Autodesk Inventor part; units mm, degrees
ref_plane "YZ Plane" through (0, 0, 0) normal (1, 0, 0) x (0, 1, 0)
ref_plane "XZ Plane" through (0, 0, 0) normal (0, 1, 0) x (-1, 0, 0)
ref_plane "XY Plane" through (0, 0, 0) normal (0, 0, 1) x (1, 0, 0)
sketch "Szkic1" plane through (0, 0, 0) normal (0, 0, 1) x (1, 0, 0)
  line L0 (0, 0) -> (50, 0) construction
  line L1 (50, 0) -> (50, 18) construction
  line L2 (50, 18) -> (0, 18) construction
  line L3 (0, 18) -> (0, 0) construction
  line L4 (25, 18) -> (25, 0) construction
  line L5 (0, 0) -> (0, 6) construction
  line L6 (0, 6) -> (50, 6) construction
  line L7 (50, 6) -> (50, 12) construction
  line L8 (50, 12) -> (0, 12) construction
  line L9 (0, 12) -> (0, 6) construction
  line L10 (0, 18) -> (10, 18) construction
  line L11 (10, 18) -> (10, 0) construction
  line L12 (50, 18) -> (30, 18) construction
  line L13 (30, 18) -> (30, 0) construction
  line L14 (40, 18) -> (40, 0) construction
  line L15 (0, 0) -> (50, 0)
  line L16 (50, 0) -> (50, 18)
  line L17 (50, 18) -> (40, 18)
  line L18 (40, 18) -> (40, 6)
  line L19 (40, 6) -> (10, 6)
  line L20 (10, 6) -> (10, 12)
  line L21 (10, 12) -> (30, 12)
  line L22 (30, 12) -> (30, 18)
  line L23 (30, 18) -> (0, 18)
  line L24 (0, 18) -> (0, 0)
  dimension "d1" = 18
  dimension "d2" = 6
  dimension "d3" = 6
  dimension "d4" = 10
  dimension "d5" = 20
  dimension "d8" = 20
extrude "Wyciągnięcie proste1" add sketch "Szkic1" along normal blind 6
properties part number "Zamkek_puszka"
Check sheet for the modelled part. Datum: model origin and axes. Units: mm. A direction names the side the tool comes from. Round coordinates to 2 decimals unless told otherwise and drop trailing zeros. Order: outer loops, then holes, each group sorted by start corner. A loop starts at its lowest first (then second) coordinate and runs counter-clockwise, first axis right, second up. Notation, with made-up numbers: (44.25, 85.25) -> (75.25, 85.25) arc R14 cw to (75.25, 107.25) -> close; hole circle Ø11 at (71.5, 35.25). An arc over 180 degrees is marked (long way). Use CSV: the item, a comma, the result in double quotes.
(1) Cross-section at B-B (z = 3.55). Record the boundary of the cut face in (x, y), and give its area (3 significant figures).
Worked out:
outline,"(0, 0) -> (50, 0) -> (50, 18) -> (40, 18) -> (40, 6) -> (10, 6) -> (10, 12) -> (30, 12) -> (30, 18) -> (0, 18) -> close"
area,"660 mm²"
(2) Draft check along X on faces 1 (the face through (50, 9, 3)), 2 (the face through (0, 9, 3)), 3 (the face through (15, 18, 3)), 4 (the face through (25, 6, 3)). Enter one of: pulls with the +X half, pulls with the -X half, needs draft (parallel to the pull), parting line crosses it, or undercut.
Worked out:
face 1,"pulls with the +X half"
face 2,"pulls with the -X half"
face 3,"needs draft"
face 4,"undercut"
(3) Cross-section at A-A (y = 13). Record the boundary of the cut face in (x, z).
Worked out:
outline,"(0, 0) -> (30, 0) -> (30, 6) -> (0, 6) -> close; (40, 0) -> (50, 0) -> (50, 6) -> (40, 6) -> close"
(4) Tool access check on faces 5 (the face through (20, 12, 3)), 6 (the face through (25, 5, 6)), 7 (the face through (30, 15, 3)). Record the directions out of +Z, -Z, +X, -X, +Y, -Y that give a thin tool (end or side, any length) a straight path to the whole face; none if there is none.
Worked out:
face 5,"+Z, -Z"
face 6,"+Z, +X, -X, +Y, -Y"
face 7,"+Z, -Z, +Y"
(5) Cross-section at C-C (x = 15). Record the boundary of the cut face in (y, z).
Worked out:
outline,"(0, 0) -> (6, 0) -> (6, 6) -> (0, 6) -> close; (12, 0) -> (18, 0) -> (18, 6) -> (12, 6) -> close"
(6) Material ranges on line 1 along X through (y, z) = (16.5, 2.1); line 2 along X through (y, z) = (9, 0.4); line 3 along Y through (x, z) = (29.5, 3.3), recorded low to high. Write a range as from..to.
Worked out:
line 1,"0..30, 40..50"
line 2,"0..10, 40..50"
line 3,"0..6, 12..18"
(7) Depth check by flat-ended pin: pin 1 (2 mm diameter, centred on x = 17.5, y = 4, fed in from -Z). Enter the tip coordinate at first touch or a pass-through.
Worked out:
pin 1,"z = 0"
